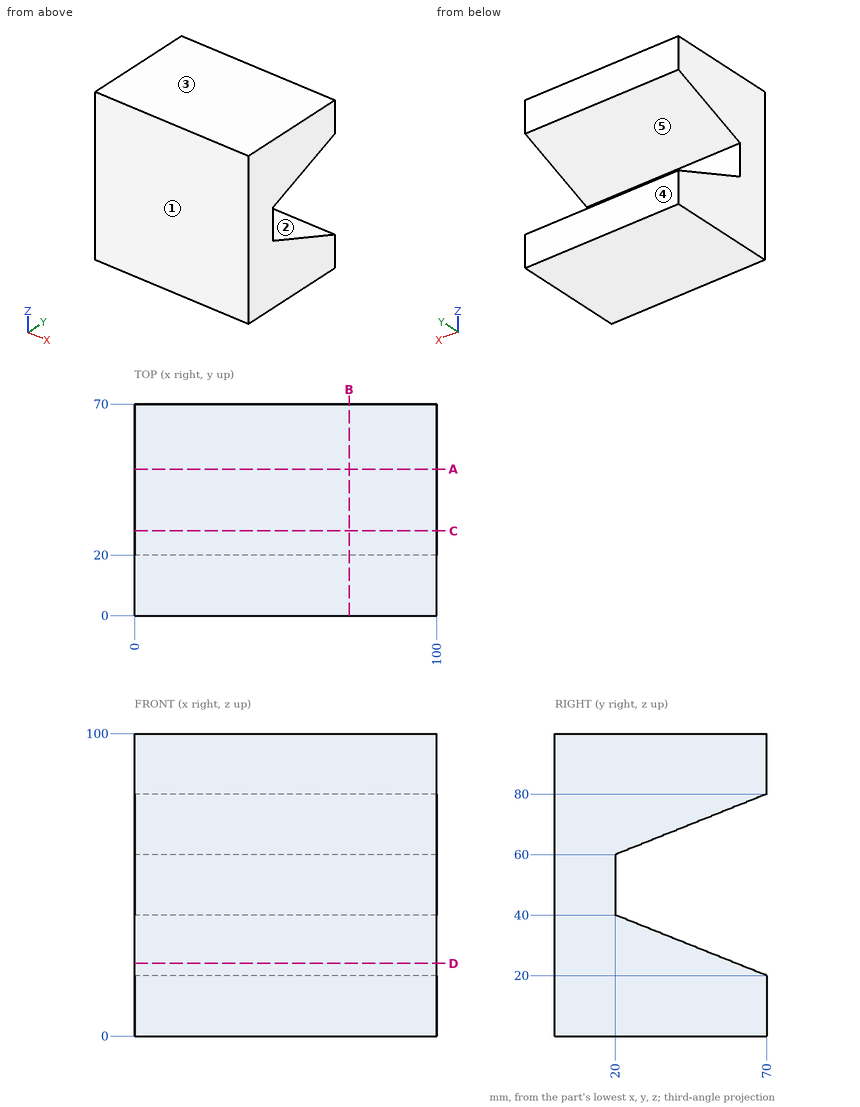
The figure shows three views and two pictorial views of one solid part (mm, origin at its lowest corner). Answer the questions. A direction names the side the tool comes from. Round coordinates to 2 decimals unless told otherwise and drop trailing zeros. Order: outer loops, then holes, each group sorted by start corner. A loop starts at its lowest first (then second) coordinate and runs counter-clockwise, first axis right, second up. Notation, with made-up numbers: (8, 48) - (35, 48) arc R30 cw to (35, 78) - close; hole circle Ø2 at (63.5, -16). An arc over 180 degrees is marked (long way). Write item = value, one per line. Start each with the question number.
1) Given pin 1 (2 mm diameter, centred on x = 34, z = 13, fed in from -Y); pin 2 (10 mm diameter, centred on x = 59.5, z = 45.5, fed in from +Y), each flat-ended and moving along its own axis, determine where each tip first touches the part or whether it passes through.
2) Section B-B, the plane x = 71 is taken. Write down the section's boundary in (y, z).
3) Straight lines are drawn through the part: L1, parallel to Y at x = 51, z = 44; L2, parallel to Z at x = 70, y = 58; L3, parallel to Z at x = 30, y = 51. For each, find the intervals that lie inside material, in ascending order.
4) Section A-A, the plane y = 48.5 is taken. Write down the section's boundary in (x, z), plus the area to 3 significant figures.
5) Section C-C, the plane y = 28 is taken. Write down the section's boundary in (x, z), plus the area to 3 significant figures.
6) For a pull along Z with two mould halves and no side action, classify the marked faces 1, 2 and 3 as released by +Z, released by -Z, zero draft, split by the parting line, or undercut.
7) Section D-D, the plane z = 24 is taken. Write down the section's boundary in (x, y).
8) For the marked faces 4 and 5, determine the directions among +Z, -Z, +X, -X, +Y, -Y from which every point of the face is accessible in a straight line to the end or side of a thin tool.
Results list:
q1.pin_1 = 0
q1.pin_2 = 20
q2.outline = (0, 0) - (70, 0) - (70, 20) - (20, 40) - (20, 60) - (70, 80) - (70, 100) - (0, 100) - close
q3.L1 = 0 to 20
q3.L2 = 0 to 24.8, 75.2 to 100
q3.L3 = 0 to 27.6, 72.4 to 100
q4.outline = (0, 0) - (100, 0) - (100, 28.6) - (0, 28.6) - close; (0, 71.4) - (100, 71.4) - (100, 100) - (0, 100) - close
q4.area = 5,720 mm^2
q5.outline = (0, 0) - (100, 0) - (100, 36.8) - (0, 36.8) - close; (0, 63.2) - (100, 63.2) - (100, 100) - (0, 100) - close
q5.area = 7,360 mm^2
q6.face_1 = zero draft
q6.face_2 = undercut
q6.face_3 = released by +Z
q7.outline = (0, 0) - (100, 0) - (100, 60) - (0, 60) - close
q8.face_4 = +Z, -Z, +X, -X, +Y
q8.face_5 = +X, -X, +Y
